Could you check a few things on this model? Use its own coordinates, in mm. A direction names the side the tool comes from. Give positions to 0.01 mm unless a question says otherwise; leave off trailing zeros. Loops run counter-clockwise (first coordinate to the right, second up) from the corner with the lowest first, then second, coordinate; pieces in that order, holes last. Notation, with made-up numbers: (-11, 36.25) - (-6, 36.25) arc R29 cw to (-6, 65.25) - close; hole circle Ø1 at (-25.5, -5). An arc over 180 degrees is marked (long way). Write each question's results on one line, items separated by ' | '. Start each with the question number.
(1) For pin 1 (1 mm diameter, centred on x = 53.5, y = 3, fed in from +Z); pin 2 (6.5 mm diameter, centred on x = 100, z = -6.13, fed in from +Y), each with a flat end and sliding along its axis, tell me the tip position at first contact or that it passes through.
(2) Suppose I cut it at C-C (x = -55.5). Please give me the cut outline in (y, z).
(3) Suppose I cut it at D-D (z = -114). Please give me the cut outline in (x, y).
(4) On a 3-axis mill with a long thin cutter (end or side, diameter ignored), from which of +Z, -Z, +X, -X, +Y, -Y can I reach the whole of each face in a straight line? I mean faces 1 (the face through (100, 5, 7.874)), 2 (the face through (-78.574, 5.07, -100.622)). Say none if no direction works.
(5) I need wall thicknesses on line 1 (X direction, y = 9.5, z = -3.5); line 2 (Z direction, x = 100, y = 6.5); line 3 (Z direction, x = 36, y = 9.75). Which ranges of each line are inside material? Lowest first, please.
(6) Suppose I cut it at B-B (y = 8.25). Please give me the cut outline in (x, z).
(7) If we mould it in two halves opening along X, with no side actions, what happens to faces 3 (the face through (120, 5, -46)), 4 (the face through (-108.59, 5.07, -130.1)), 5 (the face through (-80, 5, -44))? For each: released by +X, released by -X, zero draft, split by the parting line, or undercut.
(8) Suppose I cut it at A-A (z = -75). Please give me the cut outline in (x, y).
from build123d import *

# Parameters (mm, degrees)
SKETCH_1_R      = 2
EXTRUDE_1_DEPTH = 10
FILLET_1_R      = 40
FILLET_2_R      = 5


with BuildPart() as part:
    # 草图1 → 凸台-拉伸1 (new body)
    with BuildSketch(Plane(origin=(0, 0, 0), x_dir=(1, 0, 0), z_dir=(0, 1, 0))):
        Polygon((-120, 142.125556732), (-120, -7.874443268), (-80, -7.874443268), (-80, 102.125556732), (80, 102.125556732), (80, -7.874443268), (120, -7.874443268), (120, 142.125556732), align=None)
        with Locations(Location((-100, 97.125556732, 0), (0, 0, 270))):
            Circle(SKETCH_1_R, mode=Mode.SUBTRACT)
        with Locations(Location((100, 97.125556732, 0), (0, 0, 90))):
            Circle(SKETCH_1_R, mode=Mode.SUBTRACT)
        with Locations(Location((-100, 6.125556732, 0), (0, 0, 270))):
            Circle(SKETCH_1_R, mode=Mode.SUBTRACT)
        with Locations(Location((100, 6.125556732, 0), (0, 0, 90))):
            Circle(SKETCH_1_R, mode=Mode.SUBTRACT)
    extrude(amount=EXTRUDE_1_DEPTH)

    # 圆角1
    fillet_1_edges = [part.edges().sort_by_distance(p)[0] for p in [
        (-120, 5, -142.125556732),
        (120, 5, -142.125556732),
    ]]
    fillet(fillet_1_edges, radius=FILLET_1_R)

    # 圆角2
    fillet_2_edges = [part.edges().sort_by_distance(p)[0] for p in [
        (80, 5, -102.125556732),
        (-80, 5, -102.125556732),
    ]]
    fillet(fillet_2_edges, radius=FILLET_2_R)


solid = part.part
Output values:
1) pin 1: z = -102.13 | pin 2: y = 10
2) outline: (0, -142.13) - (10, -142.13) - (10, -102.13) - (0, -102.13) - close
3) outline: (-118.2, 0) - (118.2, 0) - (118.2, 10) - (-118.2, 10) - close
4) face 1: +Z, +X, -X, +Y, -Y | face 2: +Z, +Y, -Y
5) line 1: -120 to -80, 80 to 120 | line 2: -136.77 to -99.13, -95.13 to -8.13, -4.13 to 7.87 | line 3: -142.13 to -102.13
6) outline: (-120, -102.13) arc R40 ccw to (-80, -142.13) - (80, -142.13) arc R40 ccw to (120, -102.13) - (120, 7.87) - (80, 7.87) - (80, -97.13) arc R5 cw to (75, -102.13) - (-75, -102.13) arc R5 cw to (-80, -97.13) - (-80, 7.87) - (-120, 7.87) - close; hole circle Ø4 at (-100, -97.13); hole circle Ø4 at (-100, -6.13); hole circle Ø4 at (100, -97.13); hole circle Ø4 at (100, -6.13)
7) face 3: released by +X | face 4: released by -X | face 5: undercut
8) outline: (-120, 0) - (-80, 0) - (-80, 10) - (-120, 10) - close; (80, 0) - (120, 0) - (120, 10) - (80, 10) - close
